The listing builds one solid part. Answer for the finished solid, in the listing's coordinates (mm). Face numbers are marked on the shaded views. A direction names the side the tool comes from. Coordinates: 2 decimals unless noted, no trailing zeros. Order: outer loops, then holes, each group sorted by start corner. A loop starts at its lowest first (then second) coordinate and runs counter-clockwise, first axis right, second up. Notation, with made-up numbers: (88.25, -23) - (109.25, -23) arc R25 cw to (109.25, 14) - close; hole circle Ø7 at (-24.75, -20). An arc over 180 degrees is marked (long way). One line per item, written item: value. Start each with the question number.
```python
from build123d import *

# Parameters (mm, degrees)
PAD_DEPTH    = 38
SKETCH001_W  = 15
SKETCH001_H  = 2
PAD001_DEPTH = 26
SKETCH002_W  = 19
SKETCH002_H  = 2
PAD002_DEPTH = 10
SKETCH003_W  = 15
SKETCH003_H  = 3
POCKET_DEPTH = 40


with BuildPart() as part:
    # Sketch → Pad (new body)
    with BuildSketch(Plane.XZ):
        Polygon((0, 0), (0, 33), (13, 33), (13, 0), (10, 0), (10, 30), (3, 30), (3, 0), align=None)
    extrude(amount=PAD_DEPTH)

    # Sketch001 (on Face1 of Pad) → Pad001 (join)
    with BuildSketch(Plane(origin=(0, 0, 0), x_dir=(0, 0, -1), z_dir=(-1, 0, 0))):
        with Locations((-25.5, 37)):
            Rectangle(SKETCH001_W, SKETCH001_H)
        with Locations((-25.5, 1)):
            Rectangle(SKETCH001_W, SKETCH001_H)
    extrude(amount=PAD001_DEPTH)

    # Sketch002 (on Face7 of Pad001) → Pad002 (join)
    with BuildSketch(Plane(origin=(0, 0, 18), x_dir=(1, 0, 0), z_dir=(0, 0, -1))):
        with Locations((-16.5, 37)):
            Rectangle(SKETCH002_W, SKETCH002_H)
        with Locations((-16.5, 1)):
            Rectangle(SKETCH002_W, SKETCH002_H)
    extrude(amount=PAD002_DEPTH)

    # Sketch003 (on Face30 of Pad002) → Pocket (cut)
    with BuildSketch(Plane.XZ.offset(38)):
        with Locations((-16.5, 11.5)):
            Rectangle(SKETCH003_W, SKETCH003_H)
        with Locations((-16.5, 16.5)):
            Rectangle(SKETCH003_W, SKETCH003_H)
        with Locations((-16.5, 21.5)):
            Rectangle(SKETCH003_W, SKETCH003_H)
        with Locations((-16.5, 26.5)):
            Rectangle(SKETCH003_W, SKETCH003_H)
    extrude(amount=-POCKET_DEPTH, mode=Mode.SUBTRACT)


solid = part.part
```
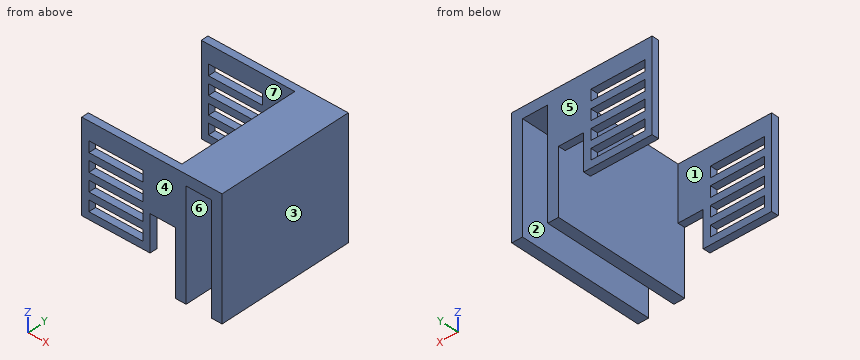
(1) For the marked faces 1, 2 and 3, determine the directions among +Z, -Z, +X, -X, +Y, -Y from which every point of the face is accessible in a straight line to the end or side of a thin tool.
(2) For a pull along Y with two mould halves and no side action, classify the marked faces 4, 5, 6 and 7 as pulls with the +Y half, pulls with the -Y half, needs draft (parallel to the pull), parting line crosses it, or undercut.
(3) Consider probe 1 along X at (y, z) = (-30, 24); probe 2 along Y at (x, z) = (-18, 9); probe 3 along Z at (x, y) = (4, -29.5). Determine where each line is inside the solid, lowest interval first.
(4) The part is cut by section A-A on z = 27. Determine the outline of the cut face in (x, y).
(5) The part is cut by section C-C on z = 4. Determine the outline of the cut face in (x, y), plus the area to 3 significant figures.
(6) The part is cut by section B-B on x = -1. Determine the outline of the cut face in (y, z).
(7) Flat-ended cylindrical pins translate along their axes: pin 1 Ø12 at (y, z) = (-20, 28.5) entering from -X; pin 2 Ø0.6 at (x, y) = (-14, -1) entering from -Z; pin 3 Ø1 at (x, y) = (6, -11) entering from -Z. Find the tip coordinate at first contact, or state that the pin passes through.
(8) The part is cut by section D-D on z = 31.5. Determine the outline of the cut face in (x, y), plus the area to 3 significant figures.
Completed:
1. face 1: +Z, -Z, -X
1. face 2: -Z, +Y, -Y
1. face 3: +Z, -Z, +X, +Y, -Y
2. face 4: pulls with the -Y half
2. face 5: pulls with the +Y half
2. face 6: needs draft
2. face 7: undercut
3. probe 1: x = 0 to 3, 10 to 13
3. probe 2: y = -38 to -36, -2 to 0
3. probe 3: z = 30 to 33
4. outline: (-26, -38) - (-24, -38) - (-24, -36) - (-26, -36) - close; (-26, -2) - (-24, -2) - (-24, 0) - (-26, 0) - close; (-9, -38) - (3, -38) - (3, 0) - (-9, 0) - (-9, -2) - (0, -2) - (0, -36) - (-9, -36) - close; (10, -38) - (13, -38) - (13, 0) - (10, 0) - close
5. outline: (0, -38) - (3, -38) - (3, 0) - (0, 0) - close; (10, -38) - (13, -38) - (13, 0) - (10, 0) - close
5. area: 228 mm2
6. outline: (-38, 18) - (-36, 18) - (-36, 33) - (-38, 33) - close; (-2, 18) - (0, 18) - (0, 33) - (-2, 33) - close
7. pin 1: stops at x = 0
7. pin 2: stops at z = 8
7. pin 3: stops at z = 30
8. outline: (-26, -38) - (13, -38) - (13, 0) - (-26, 0) - (-26, -2) - (0, -2) - (0, -36) - (-26, -36) - close
8. area: 598 mm2
